Read the model definition and answer for the solid it produces. Units are mm, in the model's axes. Coordinates: 2 decimals unless noted, no trailing zeros. Write each loop counter-clockwise with the first axis right and the second up, starting at its lowest first coordinate (ties: lowest second). Pieces come first, ordered by that corner, then holes.
(1) The mould has two halves that part along Z. Classify faces 1 (the flat face through (5, -1, -100)), 2 (the flat face through (5, -1, 95)), 3 (the flat face through (10, -1, -4)): +Z half, -Z half, draft (parallel to the pull), parting line (faces both ways), or undercut.
(2) Given pin 1 (6 mm diameter, centred on x = 8, y = 43, fed in from +Z); pin 2 (5 mm diameter, centred on y = 46.5, z = -16, fed in from -X); pin 3 (4 mm diameter, centred on x = 7.5, y = 16, fed in from +Z), each flat-ended and moving along its own axis, determine where each tip first touches the part or whether it passes through.
(3) Find the intervals of material crossed by probe 1 along Z at (x, y) = (3.25, -5.5); probe 2 along Z at (x, y) = (8.25, 22.5), in increasing order.
(4) Section B-B on x = 7.25 is taken. Write down the section's boundary in (y, z).
from build123d import *

# Parameters (mm, degrees)
F0_W     = 120
F0_H     = 200
F1_DEPTH = 10
F2_SIZE  = 9.99999


# Not quite as in the source:
# - a fillet or chamfer is up to 0.001 mm smaller than in the source, because OpenCascade refuses the exact size


with BuildPart() as f1:
    # F0 (on Right) → F1 (new body)
    with BuildSketch(Plane.YZ):
        Rectangle(F0_W, F0_H)
    extrude(amount=F1_DEPTH)

    # F2 (size 10 in the source; OpenCascade refuses exactly that, so slightly less here)
    f2_edges = [f1.edges().sort_by_distance(p)[0] for p in [
        (10, 0, 100),
    ]]
    chamfer(f2_edges, length=F2_SIZE)


solid = f1.part
Response:
1. face 1: -Z half
1. face 2: +Z half
1. face 3: draft
2. pin 1: stops at z = 95
2. pin 2: stops at x = 0
2. pin 3: stops at z = 94.5
3. probe 1: z = -100 to 96.75
3. probe 2: z = -100 to 91.75
4. outline: (-60, -100) - (60, -100) - (60, 92.75) - (-60, 92.75) - close
